Source: CAD feature listing. Evaluate the final solid. Frame: model axes, mm. A direction names the side the tool comes from. Round coordinates to 2 decimals unless told otherwise and drop trailing zeros. Loops run counter-clockwise (first coordinate to the right, second up) from the corner with the lowest first, then second, coordinate; pieces in that order, holes last. Notation, with made-up numbers: M -11.75,33.25 L 19.25,33.25 A24 ccw 19.25,62.25 Z; hole C 76.25,1 d5. An arc over 180 degrees is marked long. Write each question's results on one line, items separated by ' | '. Start each with the question number.
1. Section A-A on y = 26.5. Output: boundary loops of the cut face in (x, z), and give its area (3 significant figures).
2. Ray query, line 1 (Z direction, x = -55.5, y = 16); line 2 (X direction, y = 1.45, z = -43.4); line 3 (X direction, y = 9.5, z = 55.5). Return the intervals inside material, ascending.
3. Section D-D on y = 7.5. Give the number of separate pieces and of enclosed holes in the cut face, and give its area (3 significant figures).
4. Section C-C on z = 55.5. Output: boundary loops of the cut face in (x, y).
5. Section B-B on x = 0. Output: boundary loops of the cut face in (y, z).
6. Contact query for flat-ended pins moving along their axis: pin 1 Ø6.5 at (x, z) = (-53.99, 24.87) entering from +Y; pin 2 Ø8 at (y, z) = (5, -66.5) entering from -X; pin 3 Ø8 at (x, y) = (2, 7.5) entering from -Z. Output: stop coordinate, or through.
7. Draft query along X for faces 5 (the cylindrical face through (-70.979, 5.916, -71.445)), 6 (the flat face through (0, 2, -56)), 7 (the flat face through (60, 32, -55)). Return one class per face: released by +X, released by -X, zero draft, split by the parting line, or undercut.
8. Set-up query: faces 1 (the flat face through (80, 6, 1)), 2 (the cylindrical face through (-17.32, 6.08, 52.04)), 3 (the flat face through (-30, 7, -60)), 4 (the cylindrical face through (61.58, 23.89, -47.56)). Return all of +Z, -Z, +X, -X, +Y, -Y with unobstructed straight access to the full face (end or side cutting, diameter ignored); none if empty.
from build123d import *

# Parameters (mm, degrees)
BOSS_EXTRUDE6_DEPTH = 12
FILLET4_R           = 10
SKETCH13_R          = 4
CUT_EXTRUDE5_DEPTH  = 114.771701227
SKETCH14_R          = 10
BOSS_EXTRUDE7_DEPTH = 20
SKETCH15_R          = 4
CUT_EXTRUDE6_DEPTH  = 115.891252931
FILLET5_R           = 4
SKETCH16_R          = 11
CUT_EXTRUDE7_DEPTH  = 7
SKETCH17_R          = 1.5
CUT_EXTRUDE8_DEPTH  = 115.891252931
SKETCH18_W          = 60
SKETCH18_H          = 70
CUT_EXTRUDE9_DEPTH  = 10
FILLET6_R           = 10
SKETCH19_R          = 2.5
CUT_EXTRUDE10_DEPTH = 115.891252931


with BuildPart() as part:
    # Sketch12 → Boss-Extrude6 (new body)
    with BuildSketch(Plane(origin=(0, 0, 0), x_dir=(1, 0, 0), z_dir=(0, 1, 0))):
        with BuildLine():
            Line((-20, -50), (20, -50))
            ThreePointArc((20, -50), (28.786796564, -71.213203436), (50, -80))
            ThreePointArc((50, -80), (71.213203436, -71.213203436), (80, -50))
            Line((80, -50), (80, 50))
            ThreePointArc((80, 50), (71.213203436, 71.213203436), (50, 80))
            Line((50, 80), (-50, 80))
            ThreePointArc((-50, 80), (-71.213203436, 71.213203436), (-80, 50))
            Line((-80, 50), (-80, -50))
            ThreePointArc((-80, -50), (-71.213203436, -71.213203436), (-50, -80))
            ThreePointArc((-50, -80), (-28.786796564, -71.213203436), (-20, -50))
        make_face()
    extrude(amount=BOSS_EXTRUDE6_DEPTH)

    # Fillet4
    fillet4_edges = [part.edges().sort_by_distance(p)[0] for p in [
        (20, 6, 50),
        (-20, 6, 50),
    ]]
    fillet(fillet4_edges, radius=FILLET4_R)

    # Sketch13 → Cut-Extrude5 (cut, through all)
    with BuildSketch(Plane(origin=(0, 12, 0), x_dir=(1, 0, 0), z_dir=(0, 1, 0))):
        with Locations(Location((-55.5, 55.5, 0), (0, 0, 270))):
            Circle(SKETCH13_R)
        with Locations(Location((55.5, 55.5, 0), (0, 0, 270))):
            Circle(SKETCH13_R)
        with Locations(Location((-55.5, -55.5, 0), (0, 0, 270))):
            Circle(SKETCH13_R)
        with Locations(Location((55.5, -55.5, 0), (0, 0, 270))):
            Circle(SKETCH13_R)
    extrude(amount=-CUT_EXTRUDE5_DEPTH, mode=Mode.SUBTRACT)

    # Sketch14 → Boss-Extrude7 (add)
    with BuildSketch(Plane(origin=(0, 12, 0), x_dir=(1, 0, 0), z_dir=(0, 1, 0))):
        with Locations(Location((-55.5, 55.5, 0), (0, 0, 90))):
            Circle(SKETCH14_R)
        with Locations(Location((55.5, 55.5, 0), (0, 0, 90))):
            Circle(SKETCH14_R)
        with Locations(Location((-55.5, -55.5, 0), (0, 0, 90))):
            Circle(SKETCH14_R)
        with Locations(Location((55.5, -55.5, 0), (0, 0, 90))):
            Circle(SKETCH14_R)
    extrude(amount=BOSS_EXTRUDE7_DEPTH)

    # Sketch15 → Cut-Extrude6 (cut, through all)
    with BuildSketch(Plane.XZ.offset(-12)):
        with Locations(Location((-55.5, -55.5, 0), (0, 0, 90))):
            Circle(SKETCH15_R)
        with Locations(Location((-55.5, 55.5, 0), (0, 0, 90))):
            Circle(SKETCH15_R)
        with Locations(Location((55.5, 55.5, 0), (0, 0, 90))):
            Circle(SKETCH15_R)
        with Locations(Location((55.5, -55.5, 0), (0, 0, 90))):
            Circle(SKETCH15_R)
    extrude(amount=-CUT_EXTRUDE6_DEPTH, mode=Mode.SUBTRACT)

    # Fillet5
    fillet5_edges = [part.edges().sort_by_distance(p)[0] for p in [
        (-55.5, 12, -45.5),
        (-55.5, 12, 65.5),
        (55.5, 12, 65.5),
        (55.5, 12, -45.5),
    ]]
    fillet(fillet5_edges, radius=FILLET5_R)

    # Sketch16 → Cut-Extrude7 (cut)
    with BuildSketch(Plane(origin=(0, 12, 0), x_dir=(1, 0, 0), z_dir=(0, 1, 0))):
        with Locations(Location((0, 0, 0), (0, 0, 270))):
            Circle(SKETCH16_R)
    extrude(amount=-CUT_EXTRUDE7_DEPTH, mode=Mode.SUBTRACT)

    # Sketch17 → Cut-Extrude8 (cut, through all)
    with BuildSketch(Plane(origin=(0, 12, 0), x_dir=(1, 0, 0), z_dir=(0, 1, 0))):
        with Locations(Location((-15.5, 74.4, 0), (0, 0, 270))):
            Circle(SKETCH17_R)
        with Locations(Location((15.5, 74.4, 0), (0, 0, 270))):
            Circle(SKETCH17_R)
        with Locations(Location((-15.5, 43.4, 0), (0, 0, 270))):
            Circle(SKETCH17_R)
        with Locations(Location((15.5, 43.4, 0), (0, 0, 270))):
            Circle(SKETCH17_R)
    extrude(amount=-CUT_EXTRUDE8_DEPTH, mode=Mode.SUBTRACT)

    # Sketch18 → Cut-Extrude9 (cut)
    with BuildSketch(Plane(origin=(0, 12, 0), x_dir=(1, 0, 0), z_dir=(0, 1, 0))):
        with Locations((0, 65.9)):
            Rectangle(SKETCH18_W, SKETCH18_H)
    extrude(amount=-CUT_EXTRUDE9_DEPTH, mode=Mode.SUBTRACT)

    # Fillet6
    fillet6_edges = [part.edges().sort_by_distance(p)[0] for p in [
        (-30, 7, -30.9),
        (30, 7, -30.9),
    ]]
    fillet(fillet6_edges, radius=FILLET6_R)

    # Sketch19 → Cut-Extrude10 (cut, through all)
    with BuildSketch(Plane(origin=(0, 12, 0), x_dir=(1, 0, 0), z_dir=(0, 1, 0))):
        with Locations(Location((-53.98995062, 24.867500749, 0), (0, 0, 270))):
            Circle(SKETCH19_R)
        with Locations(Location((-53.98995062, -24.867500749, 0), (0, 0, 270))):
            Circle(SKETCH19_R)
        with Locations(Location((53.98995062, 24.867500749, 0), (0, 0, 270))):
            Circle(SKETCH19_R)
        with Locations(Location((53.98995062, -24.867500749, 0), (0, 0, 270))):
            Circle(SKETCH19_R)
    extrude(amount=-CUT_EXTRUDE10_DEPTH, mode=Mode.SUBTRACT)


solid = part.part
Taken from the geometry:
1) outline: C -55.5,-55.5 d20; C -55.5,55.5 d20; C 55.5,-55.5 d20; C 55.5,55.5 d20; hole C -55.5,-55.5 d8; hole C -55.5,55.5 d8; hole C 55.5,-55.5 d8; hole C 55.5,55.5 d8 | area: 1,060 mm^2
2) line 1: -65.5 to -59.5, -51.5 to -45.5, 45.5 to 51.5, 59.5 to 65.5 | line 2: -80 to -17, -14 to 14, 17 to 80 | line 3: -79.49 to -59.5, -51.5 to -20.2, 20.2 to 51.5, 59.5 to 79.49
3) separate pieces: 1 | enclosed holes: 9 | area: 19,700 mm^2
4) outline: M -79.49,0 L -59.5,0 L -59.5,32 L -65.5,32 L -65.5,16 A4 cw -69.5,12 L -79.49,12 Z; M -51.5,0 L -20.2,0 L -20.2,12 L -41.5,12 A4 cw -45.5,16 L -45.5,32 L -51.5,32 Z; M 20.2,0 L 51.5,0 L 51.5,32 L 45.5,32 L 45.5,16 A4 cw 41.5,12 L 20.2,12 Z; M 59.5,0 L 79.49,0 L 79.49,12 L 69.5,12 A4 cw 65.5,16 L 65.5,32 L 59.5,32 Z
5) outline: M 0,-80 L 2,-80 L 2,-30.9 L 12,-30.9 L 12,-11 L 5,-11 L 5,11 L 12,11 L 12,50 L 0,50 Z
6) pin 1: y = 12 | pin 2: x = -77.27 | pin 3: z = -30.9
7) face 5: released by -X | face 6: undercut | face 7: zero draft
8) face 1: +Z, -Z, +X, +Y, -Y | face 2: +Z, +Y, -Y | face 3: -Z, +Y | face 4: +Y
